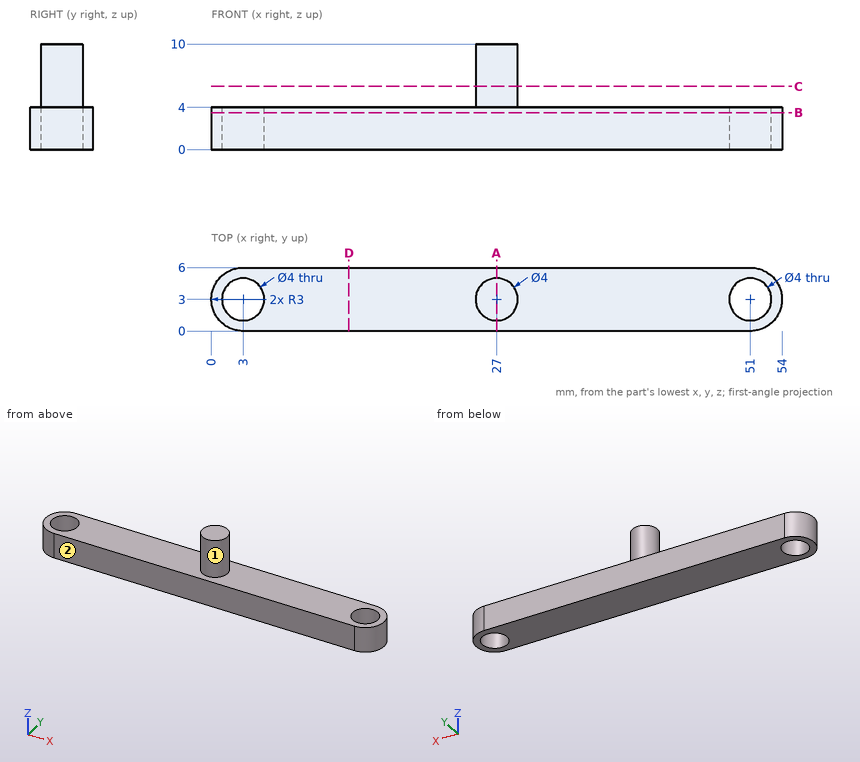
Could you check a few things on this drawing? It's one solid part, dimensions in mm from its lowest x, y, z. A direction names the side the tool comes from. Round coordinates to 2 decimals unless told otherwise and drop trailing zeros. Write each loop counter-clockwise with the first axis right and the second up, starting at its lowest first coordinate (ties: lowest second). Pieces come first, ordered by that corner, then holes. Notation, with made-up numbers: (1, 34) -> (45, 34) arc R18 ccw to (45, 69) -> close; hole circle Ø10 at (-28, 40.5). An arc over 180 degrees is marked (long way). One line per question, with ' | ' between items. Start each with the question number.
1) Suppose I cut it at C-C on z = 6. Write out the boundary of the cut face in (x, y), then the cut area to 3 significant figures.
2) I'm going to push flat-ended pins straight in: P1, Ø3, axis at x = 32.5, y = 1.5, coming from the +Z side; P2, Ø1.5, axis at y = 5, z = 2.5, coming from the -X side; P3, Ø3, axis at y = 4, z = 7.5, coming from the -X side. Where does each tip first touch, or does it pass through?
3) I need wall thicknesses on line 1 (Y direction, x = 3, z = 2.7); line 2 (X direction, y = 2.6, z = 2.75); line 3 (Z direction, x = 6.5, y = 1.7). Which ranges of each line are inside material? Lowest first, please. Write a range as [from, to].
4) Suppose I cut it at D-D on x = 13. Write out the boundary of the cut face in (y, z), then the cut area to 3 significant figures.
5) Suppose I cut it at A-A on x = 27. Write out the boundary of the cut face in (y, z).
6) Suppose I cut it at B-B on z = 3.5. Write out the boundary of the cut face in (x, y), then the cut area to 3 significant figures.
7) On a 3-axis mill with a long thin cutter (end or side, diameter ignored), from which of +Z, -Z, +X, -X, +Y, -Y can I reach the whole of each face in a straight line? I mean the marked faces 1 and 2. Say none if no direction works.
Return value:
1) outline: circle Ø4 at (27, 3) | area: 12.6 mm2
2) P1: stops at z = 4 | P2: stops at x = 0.27 | P3: stops at x = 25
3) line 1: y = [0, 1], [5, 6] | line 2: x = [0.03, 1.04], [4.96, 49.04], [52.96, 53.97] | line 3: z = [0, 4]
4) outline: (0, 0) -> (6, 0) -> (6, 4) -> (0, 4) -> close | area: 24.0 mm2
5) outline: (0, 0) -> (6, 0) -> (6, 4) -> (5, 4) -> (5, 10) -> (1, 10) -> (1, 4) -> (0, 4) -> close
6) outline: (3, 0) -> (51, 0) arc R3 ccw to (51, 6) -> (3, 6) arc R3 ccw to start; hole circle Ø4 at (3, 3); hole circle Ø4 at (51, 3) | area: 291 mm2
7) face 1: +Z | face 2: +Z, -Z, +X, -X, -Y
